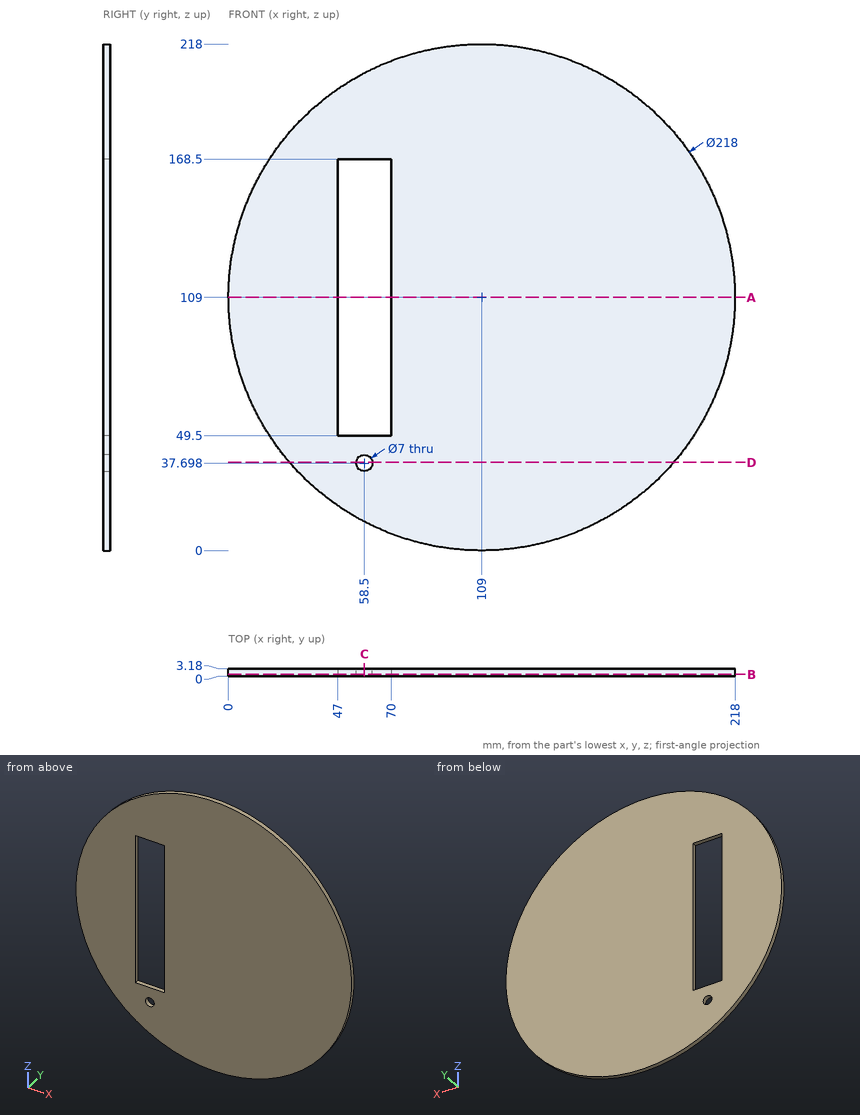
Study the drawing (mm; zero at the part's minimum x, y, z) and answer. Give positions to 0.01 mm unless a question says otherwise; leave off trailing zeros. Write each loop counter-clockwise with the first axis right and the second up, starting at its lowest first coordinate (ties: lowest second). Pieces come first, ordered by that corner, then holes. Notation, with made-up numbers: (12, -37.75) - (38, -37.75) arc R12 cw to (38, -19.75) - close; hole circle Ø8 at (45.25, 24). An arc over 180 degrees is marked (long way). Use CSV: the item, a comma, the result in double quotes. Start each with the question number.
(1) Find section C-C (x = 58.5). Give the vertices of the cut face in (y, z).
(2) Consider line 1 along X through (y, z) = (1, 68.5); line 2 along X through (y, z) = (1.6, 144); line 3 along Z through (x, y) = (53.5, 2.3). Determine where each line is inside the solid, lowest interval first.
(3) Given P1, Ø1, axis at x = 53, y = 2, coming from the +Z side; P2, Ø1.6, axis at y = 2, z = 127, coming from the -X side; P3, Ø5.5, axis at x = 58.5, z = 37.7, coming from the +Y side, each flat-ended and moving along its own axis, determine where each tip first touches the part or whether it passes through.
(4) Find section D-D (z = 38). Give the vertices of the cut face in (x, y).
(5) Find section B-B (y = 0.7). Give the vertices of the cut face in (x, z), plus the area to 4 significant figures.
(6) Find section A-A (z = 109). Give the vertices of the cut face in (x, y).
Findings below:
1,outline,"(0, 12.4) - (3.18, 12.4) - (3.18, 34.2) - (0, 34.2) - close; (0, 41.2) - (3.18, 41.2) - (3.18, 49.5) - (0, 49.5) - close; (0, 168.5) - (3.18, 168.5) - (3.18, 205.6) - (0, 205.6) - close"
2,line 1,"7.8 to 47, 70 to 210.2"
2,line 2,"5.77 to 47, 70 to 212.23"
2,line 3,"15.19 to 49.5, 168.5 to 202.81"
3,P1,"z = 202.81"
3,P2,"x = 1.37"
3,P3,"through"
4,outline,"(26.3, 0) - (55.01, 0) - (55.01, 3.18) - (26.3, 3.18) - close; (61.99, 0) - (191.7, 0) - (191.7, 3.18) - (61.99, 3.18) - close"
5,outline,"circle Ø218 at (109, 109); hole (47, 49.5) - (70, 49.5) - (70, 168.5) - (47, 168.5) - close; hole circle Ø7 at (58.5, 37.7)"
5,area,"34,550 mm2"
6,outline,"(0, 0) - (47, 0) - (47, 3.18) - (0, 3.18) - close; (70, 0) - (218, 0) - (218, 3.18) - (70, 3.18) - close"
